Verification items for the finished model (mm, model axes). Give positions to 0.01 mm unless a question says otherwise; leave off trailing zeros. Order: outer loops, then holes, each group sorted by start corner. A loop starts at its lowest first (then second) coordinate and runs counter-clockwise, first axis right, second up. Notation, with made-up numbers: (-13, 89) -> (22, 89) arc R27 ccw to (22, 120) -> close; hole circle Ø1 at (60, 70). An arc over 180 degrees is marked (long way). One line per question, with ' | ' between items. Start each with the question number.
Q1. Material ranges on probe 1 along Z at (x, y) = (0, 1.75) (3 decimals); probe 2 along Z at (x, y) = (1.25, 4); probe 3 along X at (y, z) = (5.75, -0.75), recorded low to high. Write a range as [from, to].
Q2. Mould release check, pull along X, two halves, no side actions. Record for faces 1 (the cylindrical face through (-1.38, 3.14, 6.2)), 2 (the flat face through (3, 6.35, 3)), 3 (the cylindrical face through (0.753, 3.131, 3.392)): released by +X, released by -X, zero draft, split by the parting line, or undercut.
Q3. Section check A-A on z = 0. Record the cut outline in (x, y) (3 decimals), plus the area to 3 significant figures.
Q4. Section check B-B on x = 0. Record the cut outline in (y, z) (3 decimals), plus the area to 3 significant figures.
Q5. Section check C-C on y = 1.5. Record the cut outline in (x, z) (3 decimals).
Q6. Go/stop test with flat-tipped pins: pin 1 (6 mm diameter, centred on x = -4, z = -3, fed in from -Y); pin 2 (3 mm diameter, centred on y = 1, z = -2, fed in from -X); pin 3 (1.5 mm diameter, centred on x = 1, y = 3, fed in from -Z). Record where each tip stops, or that it passes through.
from build123d import *

# Parameters (mm, degrees)
SKETCH1_R                   = 6.35
BOSS_EXTRUDE1_DEPTH         = 6.35
F_1_4_0_25_DIAMETER_HOLE1_D = 6.95000007
CHAMFER1_SIZE               = 0.508
FILLET1_R                   = 0.76


with BuildPart() as part:
    # Sketch1 → Boss-Extrude1 (new body)
    with BuildSketch(Plane(origin=(0, 0, 0), x_dir=(1, 0, 0), z_dir=(0, 1, 0))):
        Circle(SKETCH1_R)
    extrude(amount=BOSS_EXTRUDE1_DEPTH)

    # 1/4 (0.25) Diameter Hole1 (through all)
    with Locations(Plane(origin=(0, 6.35, 0), x_dir=(1, 0, 0), z_dir=(0, 1, 0))):
        with Locations((0, 0)):
            Hole(F_1_4_0_25_DIAMETER_HOLE1_D / 2)

    # Chamfer1
    chamfer1_edges = [part.edges().sort_by_distance(p)[0] for p in [
        (-6.35, 0, 0),
        (-6.35, 6.35, 0),
    ]]
    chamfer(chamfer1_edges, length=CHAMFER1_SIZE)

    # Fillet1
    fillet1_edges = [part.edges().sort_by_distance(p)[0] for p in [
        (-5.842, 0, 0),
    ]]
    fillet(fillet1_edges, radius=FILLET1_R)


solid = part.part
Filled in:
1) probe 1: [-6.35, -3.475], [3.475, 6.35] | probe 2: [-6.23, -3.24], [3.24, 6.23] | probe 3: [-6.31, -3.39], [3.39, 6.31]
2) face 1: split by the parting line | face 2: zero draft | face 3: undercut
3) outline: (-6.35, 0.508) -> (-6.065, 0.223) arc R0.76 ccw to (-5.527, 0) -> (-3.475, 0) -> (-3.475, 6.35) -> (-5.842, 6.35) -> (-6.35, 5.842) -> close; (3.475, 0) -> (5.527, 0) arc R0.76 ccw to (6.065, 0.223) -> (6.35, 0.508) -> (6.35, 5.842) -> (5.842, 6.35) -> (3.475, 6.35) -> close | area: 36.0 mm²
4) outline: (0, -5.527) arc R0.76 ccw to (0.223, -6.065) -> (0.508, -6.35) -> (5.842, -6.35) -> (6.35, -5.842) -> (6.35, -3.475) -> (0, -3.475) -> close; (0, 3.475) -> (6.35, 3.475) -> (6.35, 5.842) -> (5.842, 6.35) -> (0.508, 6.35) -> (0.223, 6.065) arc R0.76 ccw to (0, 5.527) -> close | area: 36.0 mm²
5) outline: circle Ø12.7 at (0, 0); hole circle Ø6.95 at (0, 0)
6) pin 1: y = 0 | pin 2: x = -6.33 | pin 3: z = -6.35
